Design review of the part built by this model. Coordinates are the model's own, in mm. A direction names the side the tool comes from. Coordinates: 2 decimals unless noted, no trailing zeros. Write each loop counter-clockwise with the first axis right and the second up, starting at its lowest first coordinate (ties: lowest second). Pieces come first, ordered by that corner, then holes.
Q1. Machinability: for faces 1 (the face through (1.1, 19, 23.9)), 2 (the face through (-23.2, 19, 10.3)), 3 (the face through (23.27, 21.46, -8.49)), which of the approach directions +Z, -Z, +X, -X, +Y, -Y give a long, thin tool a straight path to every point of the face, cutting with its end or side? Answer none if there is none.
Q2. Add section C-C, the plane y = 30.5. Give the boundary of the cut face in (x, z).
Q3. To check wall thickness, follow probe 1 along Z at (x, y) = (2, 23); probe 2 along X at (y, z) = (15, -8); probe 3 along Z at (x, y) = (-16.5, 15). State the ranges of each line that lie inside material, in increasing order.
Q4. Add section A-A, the plane z = 0. Give the boundary of the cut face in (x, y) (3 decimals), plus the area to 3 significant figures.
Q5. Clearance check with flat-ended pins moving along their axes: pin 1 Ø3 at (y, z) = (15, -22.5) entering from -X; pin 2 Ø6 at (x, y) = (-9, 30) entering from -Z; pin 3 Ø5.5 at (x, z) = (10, 21.5) entering from -Y. State where each tip first meets the part, or that it passes through.
Q6. Add section B-B, the plane x = 0. Give the boundary of the cut face in (y, z) (3 decimals), plus the area to 3 significant figures.
Q7. The part is to be moulded in two halves that separate along Z. For faces 4 (the face through (15.616, 30.902, -2.05)), 5 (the face through (19.52, 21.54, -19.37)), say which applies: +Z half, -Z half, draft (parallel to the pull), parting line (faces both ways), or undercut.
from build123d import *

# Parameters (mm, degrees)
SKETCH1_R                  = 15.75
BOSS_EXTRUDE1_DEPTH        = 14
SKETCH2_R                  = 29
BOSS_EXTRUDE2_DEPTH        = 10
SKETCH4_R                  = 2.5
CUT_EXTRUDE1_DEPTH         = 5
SKETCH5_R                  = 1.295
CUT_EXTRUDE2_DEPTH         = 46.19955752
CIRPATTERN1_COUNT          = 8
SKETCH6_R                  = 15.75
BOSS_EXTRUDE3_DEPTH        = 14
LOBAC_M25_THROUGH_X8_START = 14
SKETCH9_R                  = 1.3
LOBAC_M25_THROUGH_X8_DEPTH = 10
LOBAC_M25_CBORE_X8_START   = 14
SKETCH10_R                 = 2.5
LOBAC_M25_CBORE_X8_DEPTH   = 5


with BuildPart() as part:
    # Sketch1 → Boss-Extrude1 (new body)
    with BuildSketch(Plane(origin=(0, 0, 0), x_dir=(1, 0, 0), z_dir=(0, 1, 0))):
        with Locations(Location((0, 0, 0), (0, 0, 270))):
            Circle(SKETCH1_R)
    extrude(amount=BOSS_EXTRUDE1_DEPTH)

    # Sketch2 → Boss-Extrude2 (add)
    with BuildSketch(Plane(origin=(0, 14, 0), x_dir=(1, 0, 0), z_dir=(0, 1, 0))):
        with Locations(Location((0, 0, 0), (0, 0, 270))):
            Circle(SKETCH2_R)
    extrude(amount=BOSS_EXTRUDE2_DEPTH)

    # Sketch4 → Cut-Extrude1 (cut)
    with BuildSketch(Plane(origin=(0, 24, 0), x_dir=(1, 0, 0), z_dir=(0, 1, 0))):
        with Locations(Location((0, 25, 0), (0, 0, 270))):
            Circle(SKETCH4_R)
    cut_extrude1 = extrude(amount=-CUT_EXTRUDE1_DEPTH, mode=Mode.SUBTRACT)

    # Sketch5 → Cut-Extrude2 (cut, through all)
    with BuildSketch(Plane(origin=(0, 19, 0), x_dir=(1, 0, 0), z_dir=(0, 1, 0))):
        with Locations(Location((0, 25, 0), (0, 0, 270))):
            Circle(SKETCH5_R)
    cut_extrude2 = extrude(amount=-CUT_EXTRUDE2_DEPTH, mode=Mode.SUBTRACT)

    # CirPattern1: Cut-Extrude1, Cut-Extrude2 ×8 about axis
    cirpattern1_axis = Axis((0, 0, 0), (0, 1, 0))
    add([cut_extrude1.rotate(cirpattern1_axis, i * 360 / CIRPATTERN1_COUNT) for i in range(1, CIRPATTERN1_COUNT)], mode=Mode.SUBTRACT)
    add([cut_extrude2.rotate(cirpattern1_axis, i * 360 / CIRPATTERN1_COUNT) for i in range(1, CIRPATTERN1_COUNT)], mode=Mode.SUBTRACT)

    # Sketch6 → Boss-Extrude3 (add)
    with BuildSketch(Plane(origin=(0, 24, 0), x_dir=(1, 0, 0), z_dir=(0, 1, 0))):
        with Locations(Location((0, 0, 0), (0, 0, 270))):
            Circle(SKETCH6_R)
    extrude(amount=BOSS_EXTRUDE3_DEPTH)

    # Sketch9 → LoBac-M25-Through-x8 (cut)
    with BuildSketch(Plane(origin=(0, 0, 0), x_dir=(1, 0, 0), z_dir=(0, 1, 0)).offset(LOBAC_M25_THROUGH_X8_START)):
        with Locations(Location((22.17310878, -9.184402377, 0), (0, 0, 270))):
            Circle(SKETCH9_R)
        with Locations(Location((9.184402377, -22.17310878, 0), (0, 0, 270))):
            Circle(SKETCH9_R)
        with Locations(Location((-9.184402377, -22.17310878, 0), (0, 0, 270))):
            Circle(SKETCH9_R)
        with Locations(Location((-22.17310878, -9.184402377, 0), (0, 0, 270))):
            Circle(SKETCH9_R)
        with Locations(Location((-22.17310878, 9.184402377, 0), (0, 0, 270))):
            Circle(SKETCH9_R)
        with Locations(Location((-9.184402377, 22.17310878, 0), (0, 0, 270))):
            Circle(SKETCH9_R)
        with Locations(Location((9.184402377, 22.17310878, 0), (0, 0, 270))):
            Circle(SKETCH9_R)
        with Locations(Location((22.17310878, 9.184402377, 0), (0, 0, 270))):
            Circle(SKETCH9_R)
    extrude(amount=LOBAC_M25_THROUGH_X8_DEPTH, mode=Mode.SUBTRACT)

    # Sketch10 → LoBac-M25-CBore-x8 (cut)
    with BuildSketch(Plane(origin=(0, 0, 0), x_dir=(1, 0, 0), z_dir=(0, 1, 0)).offset(LOBAC_M25_CBORE_X8_START)):
        with Locations(Location((22.17310878, -9.184402377, 0), (0, 0, 270))):
            Circle(SKETCH10_R)
        with Locations(Location((9.184402377, -22.17310878, 0), (0, 0, 270))):
            Circle(SKETCH10_R)
        with Locations(Location((-9.184402377, -22.17310878, 0), (0, 0, 270))):
            Circle(SKETCH10_R)
        with Locations(Location((-22.17310878, -9.184402377, 0), (0, 0, 270))):
            Circle(SKETCH10_R)
        with Locations(Location((-22.17310878, 9.184402377, 0), (0, 0, 270))):
            Circle(SKETCH10_R)
        with Locations(Location((-9.184402377, 22.17310878, 0), (0, 0, 270))):
            Circle(SKETCH10_R)
        with Locations(Location((9.184402377, 22.17310878, 0), (0, 0, 270))):
            Circle(SKETCH10_R)
        with Locations(Location((22.17310878, 9.184402377, 0), (0, 0, 270))):
            Circle(SKETCH10_R)
    extrude(amount=LOBAC_M25_CBORE_X8_DEPTH, mode=Mode.SUBTRACT)


solid = part.part
Here are the results:
1. face 1: +Y
1. face 2: -Y
1. face 3: +Y, -Y
2. outline: circle Ø31.5 at (0, 0)
3. probe 1: z = -28.93 to -26.5, -23.5 to 23.5, 26.5 to 28.93
3. probe 2: x = -27.87 to -24.37, -19.97 to 19.97, 24.37 to 27.87
3. probe 3: z = -23.85 to -18.22, -17.14 to 17.14, 18.22 to 23.85
4. outline: (-29, 14) - (-26.295, 14) - (-26.295, 19) - (-27.5, 19) - (-27.5, 24) - (-29, 24) - close; (-23.705, 14) - (-15.75, 14) - (-15.75, 0) - (15.75, 0) - (15.75, 14) - (23.705, 14) - (23.705, 19) - (22.5, 19) - (22.5, 24) - (15.75, 24) - (15.75, 38) - (-15.75, 38) - (-15.75, 24) - (-22.5, 24) - (-22.5, 19) - (-23.705, 19) - close; (26.295, 14) - (29, 14) - (29, 24) - (27.5, 24) - (27.5, 19) - (26.295, 19) - close
4. area: 1,390 mm2
5. pin 1: stops at x = -20
5. pin 2: stops at z = -14.56
5. pin 3: stops at y = 14
6. outline: (0, -15.75) - (14, -15.75) - (14, -23.705) - (19, -23.705) - (19, -22.5) - (24, -22.5) - (24, -15.75) - (38, -15.75) - (38, 15.75) - (24, 15.75) - (24, 22.5) - (19, 22.5) - (19, 23.705) - (14, 23.705) - (14, 15.75) - (0, 15.75) - close; (14, -29) - (24, -29) - (24, -27.5) - (19, -27.5) - (19, -26.295) - (14, -26.295) - close; (14, 26.295) - (19, 26.295) - (19, 27.5) - (24, 27.5) - (24, 29) - (14, 29) - close
6. area: 1,390 mm2
7. face 4: parting line
7. face 5: undercut
